from build123d import *

# Parameters (mm, degrees)
F0_W     = 50
F0_H     = 15
F1_DEPTH = 2
F2_R     = 3
F3_R     = 5
F4_R     = 5


with BuildPart() as f1:
    # F0 (on Top) → F1 (new body)
    with BuildSketch(Plane.XY):
        with Locations((-25, 7.5)):
            Rectangle(F0_W, F0_H)
    extrude(amount=F1_DEPTH)

    # F2
    f2_edges = [f1.edges().sort_by_distance(p)[0] for p in [
        (0, 15, 1),
    ]]
    fillet(f2_edges, radius=F2_R)

    # F3
    f3_edges = [f1.edges().sort_by_distance(p)[0] for p in [
        (0, 0, 1),
    ]]
    fillet(f3_edges, radius=F3_R)

    # F4
    f4_edges = [f1.edges().sort_by_distance(p)[0] for p in [
        (-50, 15, 1),
        (-50, 0, 1),
    ]]
    fillet(f4_edges, radius=F4_R)


solid = f1.part
Check sheet for the modelled part. Datum: model origin and axes. Units: mm. Give positions to 0.01 mm unless a question says otherwise; leave off trailing zeros. Write each loop counter-clockwise with the first axis right and the second up, starting at its lowest first coordinate (ties: lowest second). Pieces come first, ordered by that corner, then holes. Notation, with made-up numbers: (86.5, 72.5) -> (108.5, 72.5) arc R24 ccw to (108.5, 94.5) -> close; hole circle Ø2 at (41.5, 16.5). An arc over 180 degrees is marked (long way). One line per item, written item: value. Start each with the question number.
Item 1: Section check A-A on z = 0.9. Record the cut outline in (x, y), then the cut area to 3 significant figures.
Item 2: Material ranges on probe 1 along Y at (x, z) = (-4, 0.65); probe 2 along X at (y, z) = (4.25, 1.9); probe 3 along X at (y, z) = (13.75, 0.45), recorded low to high. Write a range as from..to.
Item 3: Gauge pin test, flat end, axial feed: pin 1 (1 mm diameter, centred on y = 4, z = 1.5, fed in from +X). Record the tip position at first contact, or that the pin passes through.
Item 4: Section check B-B on y = 1.75. Record the cut outline in (x, z), then the cut area to 3 significant figures.
Results list:
1. outline: (-50, 5) arc R5 ccw to (-45, 0) -> (-5, 0) arc R5 ccw to (0, 5) -> (0, 12) arc R3 ccw to (-3, 15) -> (-45, 15) arc R5 ccw to (-50, 10) -> close
1. area: 732 mm²
2. probe 1: 0.1..15
2. probe 2: -49.94..-0.06
2. probe 3: -48.31..-0.56
3. pin 1: x = -0.03
4. outline: (-48.8, 0) -> (-1.2, 0) -> (-1.2, 2) -> (-48.8, 2) -> close
4. area: 95.2 mm²
